Job drawing, mm, ordinate dimensions from the low corner. One solid piece. Round coordinates to 2 decimals unless told otherwise and drop trailing zeros. Loops run counter-clockwise (first coordinate to the right, second up) from the corner with the lowest first, then second, coordinate; pieces in that order, holes last.
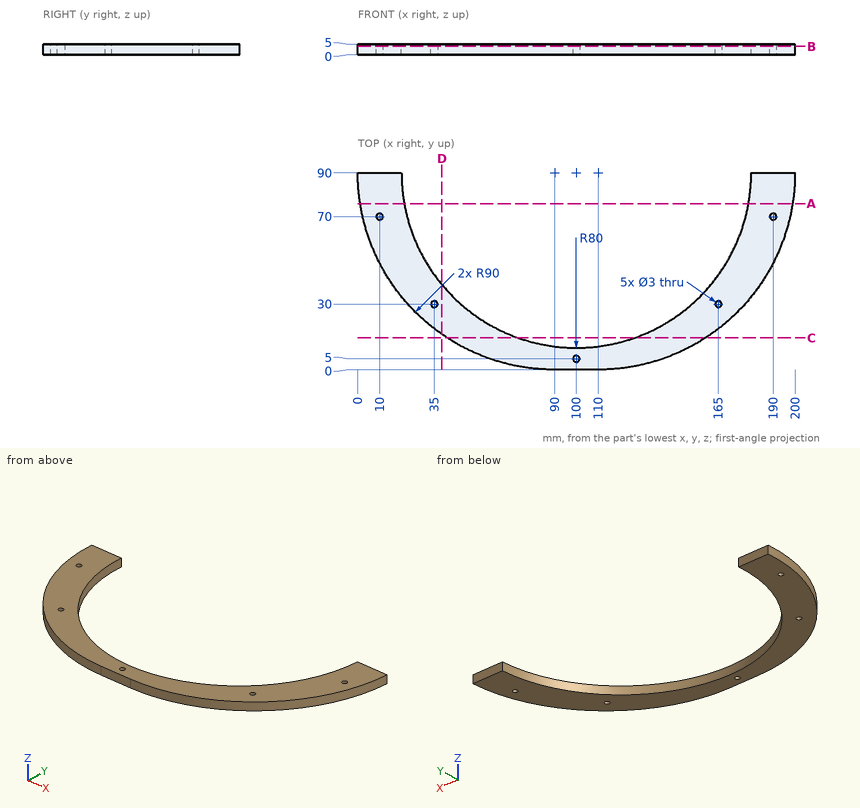
1) Slice it at B-B, the plane z = 3.95. Give the cut face in (x, y).
Values:
outline: (0, 90) arc R90 ccw to (90, 0) - (110, 0) arc R90 ccw to (200, 90) - (180, 90) arc R80 cw to (20, 90) - close; hole circle Ø3 at (10, 70); hole circle Ø3 at (35, 30); hole circle Ø3 at (100, 5); hole circle Ø3 at (165, 30); hole circle Ø3 at (190, 70)
2) Slice it at C-C, the plane y = 14.5. Give the cut face in (x, z), then the cut area to 3 significant figures.
Values:
outline: (41.01, 0) - (73.55, 0) - (73.55, 5) - (41.01, 5) - close; (126.45, 0) - (158.99, 0) - (158.99, 5) - (126.45, 5) - close
area: 325 mm2
3) Slice it at A-A, the plane y = 76. Give the cut face in (x, z).
Values:
outline: (1.1, 0) - (21.23, 0) - (21.23, 5) - (1.1, 5) - close; (178.77, 0) - (198.9, 0) - (198.9, 5) - (178.77, 5) - close
4) Wall check: line 1 along X through (y, z) = (30, 2.85); line 2 along Y through (x, z) = (100, 2.9); line 3 along X through (y, z) = (70, 3.15). Give the ranges that are in metal, low to high.
Values:
line 1: x = 22.92 to 33.5, 36.5 to 47.08, 152.92 to 163.5, 166.5 to 177.08
line 2: y = 0 to 3.5, 6.5 to 10
line 3: x = 2.25 to 8.5, 11.5 to 22.54, 177.46 to 188.5, 191.5 to 197.75
5) Slice it at D-D, the plane x = 38.5. Give the cut face in (y, z), then the cut area to 3 significant figures.
Values:
outline: (16.19, 0) - (38.84, 0) - (38.84, 5) - (16.19, 5) - close
area: 113 mm2
6) Drop flat-ended pins along their axis: pin 1 Ø1.5 at (x, z) = (134, 0.5) entering from +Y; pin 2 Ø2 at (x, z) = (171.5, 0.5) entering from +Y; pin 3 Ø2 at (y, z) = (50.5, 1) entering from -X; pin 4 Ø5 at (x, y) = (10, 70) entering from -Z. Give the stop position or say it passes through.
Values:
pin 1: stops at y = 17.94
pin 2: stops at y = 56.18
pin 3: stops at x = 8.65
pin 4: stops at z = 0
